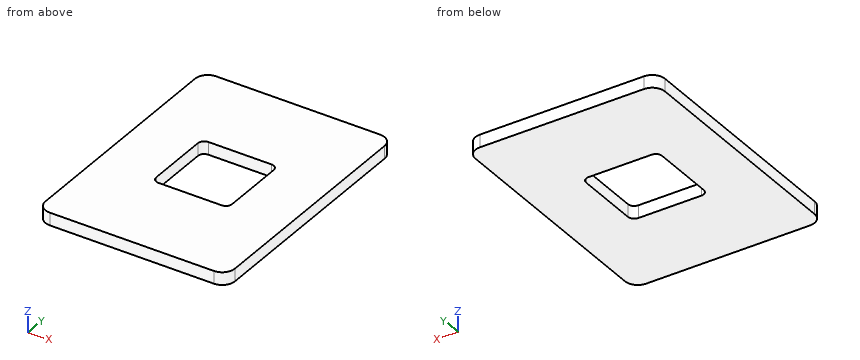
from build123d import *

# Parameters (mm, degrees)
ESQUISSE1_W             = 30
ESQUISSE1_H             = 40
BOSS_EXTRU_1_DEPTH      = 2
CONG_1_R                = 2
ESQUISSE3_W             = 12
ESQUISSE3_H             = 12
ENL_V_MAT_EXTRU_1_DEPTH = 10
CONG_2_R                = 1


with BuildPart() as part:
    # Esquisse1 → Boss.-Extru.1 (new body)
    with BuildSketch(Plane.XY):
        Rectangle(ESQUISSE1_W, ESQUISSE1_H)
    extrude(amount=BOSS_EXTRU_1_DEPTH)

    # Congé1
    cong_1_edges = [part.edges().sort_by_distance(p)[0] for p in [
        (15, -20, 1),
        (-15, -20, 1),
        (-15, 20, 1),
        (15, 20, 1),
    ]]
    fillet(cong_1_edges, radius=CONG_1_R)

    # Esquisse3 → Enlèv. mat.-Extru.1 (cut)
    with BuildSketch(Plane(origin=(0, 0, 0), x_dir=(-1, 0, 0), z_dir=(0, 0, -1))):
        Rectangle(ESQUISSE3_W, ESQUISSE3_H)
    extrude(amount=-ENL_V_MAT_EXTRU_1_DEPTH, mode=Mode.SUBTRACT)

    # Congé2
    cong_2_edges = [part.edges().sort_by_distance(p)[0] for p in [
        (-6, 6, 1),
        (-6, -6, 1),
        (6, -6, 1),
        (6, 6, 1),
    ]]
    fillet(cong_2_edges, radius=CONG_2_R)


solid = part.part
The listing builds one solid part. Answer for the finished solid, in the listing's coordinates (mm). Coordinates: 2 decimals unless noted, no trailing zeros. Order: outer loops, then holes, each group sorted by start corner. A loop starts at its lowest first (then second) coordinate and runs counter-clockwise, first axis right, second up. Notation, with made-up numbers: M 44.25,50 L 93.25,50 A12 ccw 93.25,56 Z; hole C 31.25,-12 d2. An arc over 180 degrees is marked long. Use CSV: the item, a comma, the result in double quotes.
Q1. Straight lines are drawn through the part: L1, parallel to Y at x = 1.5, z = 1.5; L2, parallel to X at y = 0.5, z = 0.35. For each, find the intervals that lie inside material, in ascending order.
Here are the results:
L1,"-20 to -6, 6 to 20"
L2,"-15 to -6, 6 to 15"
Q2. Section A-A (y = -1) is taken. Determine the outline of the cut face in (x, z), then the cut area to 3 significant figures.
Here are the results:
outline,"M -15,0 L -6,0 L -6,2 L -15,2 Z; M 6,0 L 15,0 L 15,2 L 6,2 Z"
area,"36.0 mm2"
Q3. Section B-B (x = -0.75) is taken. Determine the outline of the cut face in (y, z).
Here are the results:
outline,"M -20,0 L -6,0 L -6,2 L -20,2 Z; M 6,0 L 20,0 L 20,2 L 6,2 Z"
Q4. Section C-C (z = 0.65) is taken. Determine the outline of the cut face in (x, y), then the cut area to 3 significant figures.
Here are the results:
outline,"M -15,-18 A2 ccw -13,-20 L 13,-20 A2 ccw 15,-18 L 15,18 A2 ccw 13,20 L -13,20 A2 ccw -15,18 Z; hole M -6,-5 A1 ccw -5,-6 L 5,-6 A1 ccw 6,-5 L 6,5 A1 ccw 5,6 L -5,6 A1 ccw -6,5 Z"
area,"1,050 mm2"
